Could you check a few things on this model? Use its own coordinates, in mm. Face numbers are marked on the shaded views. A direction names the side the tool comes from. Coordinates: 2 decimals unless noted, no trailing zeros. Write each loop counter-clockwise with the first axis right and the second up, starting at its lowest first coordinate (ties: lowest second). Pieces come first, ordered by that corner, then holes. Notation, with made-up numbers: (24, -19) - (64, -19) arc R12 cw to (64, -2) - close; hole circle Ø4 at (-18, 45). An arc over 180 degrees is marked (long way). Answer as a JSON object with one key per item and string values. Group by question number.
1) Will these pins go through, and if not, where does the flat tip stop? pin 1 Ø5 at (y, z) = (-3, 5) entering from +X; pin 2 Ø1.5 at (y, z) = (1.5, 1.5) entering from +X.
2) If we section it at A-A (y = 0): Write out the boundary of the cut face in (x, z), plus the area to 3 significant figures.
3) On a 3-axis mill with a long thin cutter (end or side, diameter ignored), from which of +Z, -Z, +X, -X, +Y, -Y can I reach the whole of each face in a straight line? I mean the marked faces 1 and 2. Say none if no direction works.
4) Please list where these lines run through material, in increasing order: line 1 along X through (y, z) = (0, 5.5); line 2 along X through (y, z) = (0, 8).
5) If we section it at D-D (z = 2.5): Write out the boundary of the cut face in (x, y).
6) We'd pull the mould along Y, two halves only. Please class the marked faces 3, 4 and 5: released by +Y, released by -Y, zero draft, split by the parting line, or undercut.
7) If we section it at B-B (z = 5.5): Write out the boundary of the cut face in (x, y), plus the area to 3 significant figures.
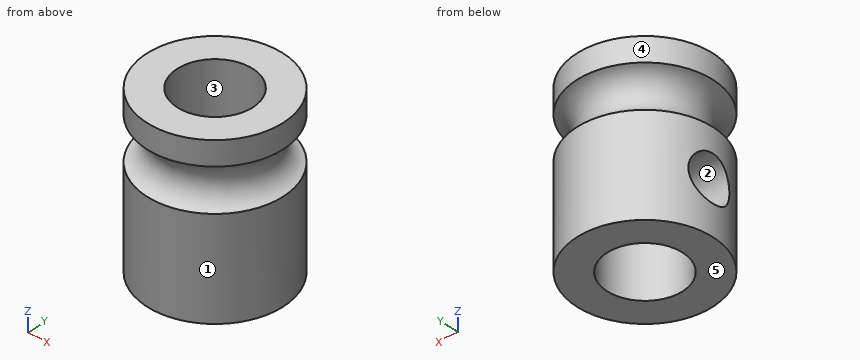
Autodesk Inventor part; units mm, degrees
ref_plane "Work Plane1" through (-4.5, 0, 0) normal (1, 0, 0) x (0, 1, 0)
ref_plane "XZ Plane" through (0, 0, 0) normal (0, 1, 0) x (-1, 0, 0)
ref_plane "XY Plane" through (0, 0, 0) normal (0, 0, 1) x (1, 0, 0)
sketch "Sketch1" plane through (0, 0, 0) normal (0, 0, 1) x (1, 0, 0)
  circle A0 centre (0, 0) radius 4.5
  dimension "d0" = 9
extrude "Extrusion1" add sketch "Sketch1" along normal blind 11
sketch "Sketch2" plane through (0, 0, 11) normal (0, 0, 1) x (1, 0, 0)
  circle A0 centre (0, 0) radius 4.5
  circle A1 centre (0, 0) radius 2.5
  dimension "d3" = 5
extrude "Extrusion2" cut sketch "Sketch2" against normal up to next contours A1
ref_plane "Work Plane1" through (-4.5, 0, 0) normal (1, 0, 0) x (0, 1, 0)
sketch "Sketch3" plane through (-4.5, 0, 0) normal (1, 0, 0) x (0, 1, 0)
  circle A0 centre (0, 3.5) radius 1.5
  point P0 (0, 0)
  dimension "d6" = 3.5
  dimension "d7" = 3
extrude "Extrusion3" cut sketch "Sketch3" along normal up to next
thread "Thread1"
sketch "Sketch4" plane through (0, 0, 0) normal (0, 1, 0) x (-1, 0, 0)
  line L0 (4.5, 0) -> (4.5, 11)
  circle A0 centre (5, 8) radius 1.5
  line L1 (0, 13.2) -> (0, -2.2)
  point P0 (0, 0)
  dimension "d12" = 3
  dimension "d13" = 0.5
  dimension "d14" = 8
revolve "Revolution1" cut sketch "Sketch4" angle 360 about axis through (0, 0, 11) along (0, 0, -1)
equation "\"d8\" = d7"
properties part number "DriveGearMK8" material "Aluminum 6061"
Here are the results:
{
 "1": {"pin 1": "stops at x = 4.47", "pin 2": "stops at x = 4.44"},
 "2": {"outline": "(-4.5, 0) - (-2.5, 0) - (-2.5, 2) - (-4.5, 2) - close; (-4.5, 5) - (-2.5, 5) - (-2.5, 11) - (-4.5, 11) - (-4.5, 9.41) arc R1.5 cw to (-4.5, 6.59) - close; (2.5, 0) - (4.5, 0) - (4.5, 6.59) arc R1.5 cw to (4.5, 9.41) - (4.5, 11) - (2.5, 11) - close", "area": "33.9 mm²"},
 "3": {"face 1": "+Z, -Z", "face 2": "-X"},
 "4": {"line 1": "x = -4.5 to -2.5, 2.5 to 4.5", "line 2": "x = -3.5 to -2.5, 2.5 to 3.5"},
 "5": {"outline": "(-4.36, -1.12) arc R4.5 ccw (long way) to (-4.36, 1.12) - (-2.24, 1.12) arc R2.5 cw (long way) to (-2.24, -1.12) - close"},
 "6": {"face 3": "undercut", "face 4": "split by the parting line", "face 5": "zero draft"},
 "7": {"outline": "circle Ø9 at (0, 0); hole circle Ø5 at (0, 0)", "area": "44.0 mm²"}
}
